Can you work these out from the drawing? Everything is in mm from the part's minimum corner. Round coordinates to 2 decimals unless told otherwise and drop trailing zeros. Write each loop counter-clockwise with the first axis right and the second up, starting at its lowest first coordinate (ties: lowest second). Pieces come first, ordered by that corner, then holes. Notation, with made-up numbers: M 43.25,-38 L 66.25,-38 A9 ccw 66.25,-21 Z; hole C 66,6.25 d2. An arc over 180 degrees is marked long. Use one line per item in the form item = value. Start each with the question number.
Q1. I want a section at B-B on z = 3.25. List the corners of the cut face in (x, y) for me.
Q2. I want a section at C-C on x = 89.5. List the corners of the cut face in (y, z) for me, and give its area (3 significant figures).
Q3. I want a section at A-A on y = 34.5. List the corners of the cut face in (x, z) for me.
Q4. I'm going to push a flat-ended pin straight in: pin 1 Ø1 at (x, y) = (78.5, 39) entering from -Z. Where does the tip first touch, or does it pass through?
Q5. I need wall thicknesses on line 1 along Z through (x, y) = (79.5, 11.5); line 2 along Z through (x, y) = (75.5, 39). Which ranges of each line are inside material? Lowest first, please. Write a range as from..to.
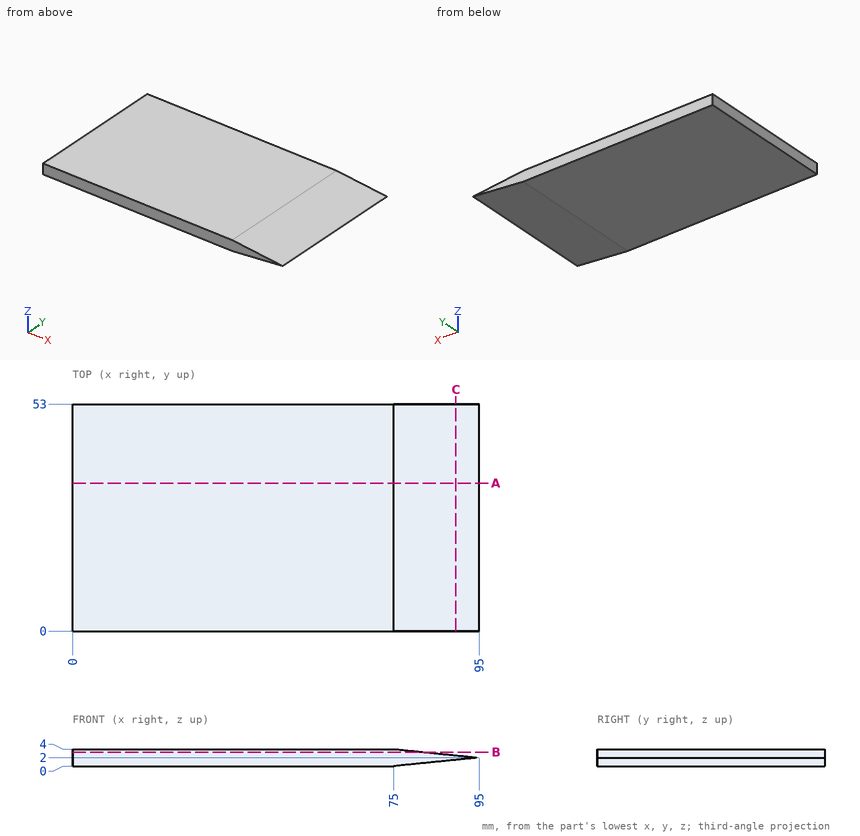
Reported:
q1.outline = M 0,0 L 82.5,0 L 82.5,53 L 0,53 Z
q2.outline = M 0,1.45 L 53,1.45 L 53,2.55 L 0,2.55 Z
q2.area = 58.3 mm^2
q3.outline = M 0,0 L 75,0 L 95,2 L 75,4 L 0,4 Z
q4.pin_1 = 0.3
q5.line_1 = 0.45..3.55
q5.line_2 = 0.05..3.95
